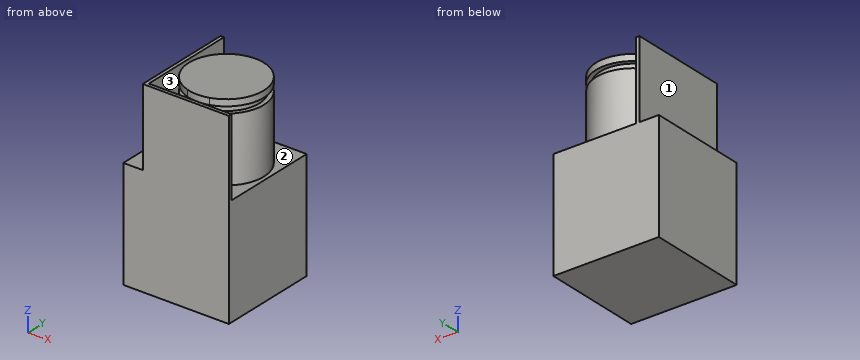
from build123d import *

# Parameters (mm, degrees)
SKETCH1_W           = 49
SKETCH1_H           = 46.6
BOSS_EXTRUDE1_DEPTH = 51
BOSS_EXTRUDE2_DEPTH = 36
BOSS_EXTRUDE3_DEPTH = 36
CUT_EXTRUDE1_START  = -3
SKETCH4_R           = 17.444416191
SKETCH4_R_2         = 15.444416191
CUT_EXTRUDE1_DEPTH  = 3
CUT_EXTRUDE2_DEPTH  = 6


with BuildPart() as part:
    # Sketch1 → Boss-Extrude1 (new body)
    with BuildSketch(Plane.XY):
        Rectangle(SKETCH1_W, SKETCH1_H)
    extrude(amount=BOSS_EXTRUDE1_DEPTH)

    # Sketch2 → Boss-Extrude2 (add)
    with BuildSketch(Plane.XY.offset(51)):
        Polygon((24.5, -23.3), (24.5, -21.7125), (-13.9125, -21.7125), (-13.9125, 23.3), (-15.5, 23.3), (-15.5, -23.3), align=None)
    extrude(amount=BOSS_EXTRUDE2_DEPTH)

    # Sketch3 → Boss-Extrude3 (add)
    with BuildSketch(Plane.XY.offset(51)):
        with BuildLine():
            Line((0.29375, -21.7125), (0.29375, -16.7125))
            ThreePointArc((0.29375, -16.7125), (5.29375, 17.444416191), (10.29375, -16.7125))
            Line((10.29375, -16.7125), (10.29375, -21.7125))
            Line((10.29375, -21.7125), (0.29375, -21.7125))
        make_face()
    extrude(amount=BOSS_EXTRUDE3_DEPTH)

    # Sketch4 → Cut-Extrude1 (cut)
    with BuildSketch(Plane.XY.offset(87).offset(CUT_EXTRUDE1_START)):
        with Locations((5.29375, 0)):
            Circle(SKETCH4_R)
        with Locations((5.29375, 0)):
            Circle(SKETCH4_R_2, mode=Mode.SUBTRACT)
    extrude(amount=-CUT_EXTRUDE1_DEPTH, mode=Mode.SUBTRACT)

    # Sketch5 → Cut-Extrude2 (cut)
    with BuildSketch(Plane.XY.offset(87)):
        with BuildLine():
            Line((0.29375, -21.7125), (10.29375, -21.7125))
            Line((10.29375, -21.7125), (10.29375, -16.7125))
            ThreePointArc((10.29375, -16.7125), (5.29375, -17.444416191), (0.29375, -16.7125))
            Line((0.29375, -16.7125), (0.29375, -21.7125))
        make_face()
    extrude(amount=-CUT_EXTRUDE2_DEPTH, mode=Mode.SUBTRACT)


solid = part.part
Here's how the part is built. I have some questions about the finished solid (model axes, mm). Face numbers are marked on the shaded views. A direction names the side the tool comes from. Give positions to 0.01 mm unless a question says otherwise; leave off trailing zeros. Loops run counter-clockwise (first coordinate to the right, second up) from the corner with the lowest first, then second, coordinate; pieces in that order, holes last. Notation, with made-up numbers: (25.5, -15) -> (82.5, -15) arc R7 ccw to (82.5, -7) -> close; hole circle Ø11 at (48, 39). An arc over 180 degrees is marked (long way). One line per item, written item: value.
Q1. On a 3-axis mill with a long thin cutter (end or side, diameter ignored), from which of +Z, -Z, +X, -X, +Y, -Y can I reach the whole of each face in a straight line? I mean the marked faces 1, 2 and 3. Say none if no direction works.
Answers follow:
face 1: +Z, -X, +Y, -Y
face 2: +Z
face 3: +Z, +Y
Q2. Suppose I cut it at C-C on y = 0. Please give me the cut outline in (x, z), then the cut area to 3 significant figures.
Answers follow:
outline: (-24.5, 0) -> (24.5, 0) -> (24.5, 51) -> (22.74, 51) -> (22.74, 81) -> (20.74, 81) -> (20.74, 84) -> (22.74, 84) -> (22.74, 87) -> (-12.15, 87) -> (-12.15, 84) -> (-10.15, 84) -> (-10.15, 81) -> (-12.15, 81) -> (-12.15, 51) -> (-13.91, 51) -> (-13.91, 87) -> (-15.5, 87) -> (-15.5, 51) -> (-24.5, 51) -> close
area: 3,800 mm^2
Q3. Suppose I cut it at B-B on y = 16.5. Please give me the cut outline in (x, z).
Answers follow:
outline: (-24.5, 0) -> (24.5, 0) -> (24.5, 51) -> (10.96, 51) -> (10.96, 81) -> (-0.37, 81) -> (-0.37, 51) -> (-13.91, 51) -> (-13.91, 87) -> (-15.5, 87) -> (-15.5, 51) -> (-24.5, 51) -> close; (-0.37, 84) -> (10.96, 84) -> (10.96, 87) -> (-0.37, 87) -> close
Q4. I'm going to push flat-ended pins straight in: pin 1 Ø4 at (y, z) = (-12.5, 68.5) entering from -X; pin 2 Ø11 at (x, z) = (5, 68.5) entering from +Y; pin 3 Ø3 at (y, z) = (-4.5, 57.5) entering from +X; pin 4 Ø7 at (x, y) = (-18, 7) entering from +Z. Where does each tip first touch, or does it pass through?
Answers follow:
pin 1: x = -15.5
pin 2: y = 17.44
pin 3: x = 22.48
pin 4: z = 87
Q5. If I drill on line 1 along Z through (x, y) = (-9, 7); line 2 along Z through (x, y) = (10, 20.5); line 3 along Y through (x, z) = (-7, 79), over which ranges is the centre line in solid material (lowest first)?
Answers follow:
line 1: 0 to 81, 84 to 87
line 2: 0 to 51
line 3: -23.3 to -21.71, -12.38 to 12.38
Q6. Suppose I cut it at D-D on x = -5.5. Please give me the cut outline in (y, z).
Answers follow:
outline: (-23.3, 0) -> (23.3, 0) -> (23.3, 51) -> (13.7, 51) -> (13.7, 81) -> (11.05, 81) -> (11.05, 84) -> (13.7, 84) -> (13.7, 87) -> (-13.7, 87) -> (-13.7, 84) -> (-11.05, 84) -> (-11.05, 81) -> (-13.7, 81) -> (-13.7, 51) -> (-21.71, 51) -> (-21.71, 87) -> (-23.3, 87) -> close
Q7. Suppose I cut it at A-A on z = 75. Please give me the cut outline in (x, y).
Answers follow:
outline: (-15.5, -23.3) -> (24.5, -23.3) -> (24.5, -21.71) -> (10.29, -21.71) -> (10.29, -16.71) arc R17.44 ccw (long way) to (0.29, -16.71) -> (0.29, -21.71) -> (-13.91, -21.71) -> (-13.91, 23.3) -> (-15.5, 23.3) -> close
